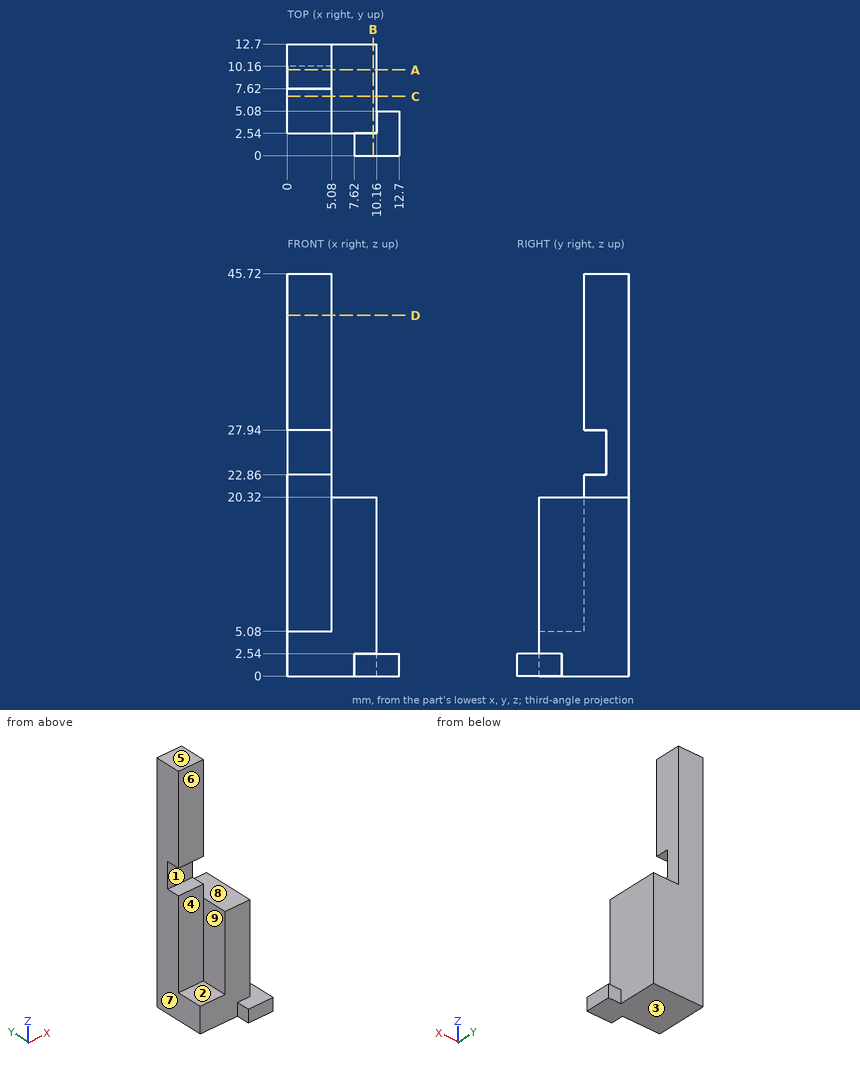
Answer from the drawing. Dimensions are ordinates in mm from the lowest x, y and z of the part. A direction names the side the tool comes from. Round coordinates to 2 decimals unless told otherwise and drop trailing zeros. Loops run counter-clockwise (first coordinate to the right, second up) from the corner with the lowest first, then second, coordinate; pieces in that order, holes last. Notation, with made-up numbers: (13.5, -1.75) - (53.5, -1.75) arc R4 ccw to (53.5, 2.25) - close; hole circle Ø5 at (20.25, -31). An arc over 180 degrees is marked (long way). Return JSON: item names as keys, results as strings. Group by question number.
1. Which of the six approach directions +Z, -Z, +X, -X, +Y, -Y give full straight-line access (tool end or side, diameter ignored) to the marked faces 5, 6, 7, 8 and 9?
2. The part is cut by section D-D on z = 41. Determine the outline of the cut face in (x, y), then the cut area to 3 significant figures.
3. The part is cut by section B-B on x = 9.75. Determine the outline of the cut face in (y, z).
4. Each of these flat-tipped pins is pushed along its axis until it touches: P1, Ø5, axis at x = 7, z = 9, coming from the -Y side; P2, Ø5.5, axis at x = 3, z = 25.5, coming from the -Y side; P3, Ø0.8, axis at x = 11.5, z = 2, coming from the +Y side. Where does it stop, or does it pass through?
5. Consider probe 1 along Z at (x, y) = (2.25, 8.5); probe 2 along Y at (x, z) = (7.5, 7.5); probe 3 along Z at (x, y) = (3, 5.5). Determine where each line is inside the solid, lowest interval first.
6. The mould has two halves that part along Z. Classify the marked faces 1, 2, 3 and 4: pulls with the +Z half, pulls with the -Z half, needs draft (parallel to the pull), parting line crosses it, or undercut.
7. The part is cut by section C-C on y = 6.75. Determine the outline of the cut face in (x, z).
8. The part is cut by section A-A on y = 9.75. Determine the outline of the cut face in (x, z).
Resolved:
{
 "1": {"face 5": "+Z, +X, -X, +Y, -Y", "face 6": "+Z, +X, -X, -Y", "face 7": "+Z, -Z, -X, +Y, -Y", "face 8": "+Z, +X, +Y, -Y", "face 9": "+Z, -X, -Y"},
 "2": {"outline": "(0, 7.62) - (5.08, 7.62) - (5.08, 12.7) - (0, 12.7) - close", "area": "25.8 mm²"},
 "3": {"outline": "(0, 0) - (12.7, 0) - (12.7, 20.32) - (2.54, 20.32) - (2.54, 2.54) - (0, 2.54) - close"},
 "4": {"P1": "stops at y = 2.54", "P2": "stops at y = 7.62", "P3": "stops at y = 5.08"},
 "5": {"probe 1": "z = 0 to 22.86, 27.94 to 45.72", "probe 2": "y = 2.54 to 12.7", "probe 3": "z = 0 to 5.08"},
 "6": {"face 1": "undercut", "face 2": "pulls with the +Z half", "face 3": "pulls with the -Z half", "face 4": "needs draft"},
 "7": {"outline": "(0, 0) - (10.16, 0) - (10.16, 20.32) - (5.08, 20.32) - (5.08, 5.08) - (0, 5.08) - close"},
 "8": {"outline": "(0, 0) - (10.16, 0) - (10.16, 20.32) - (5.08, 20.32) - (5.08, 22.86) - (0, 22.86) - close; (0, 27.94) - (5.08, 27.94) - (5.08, 45.72) - (0, 45.72) - close"}
}
